For this review, take the finished solid that the model builds, in its own axes (mm). Give positions to 0.01 mm unless a question says otherwise; leave off trailing zeros. Order: outer loops, then holes, each group sorted by start corner. A loop starts at its lowest first (then second) coordinate and runs counter-clockwise, first axis right, second up. Notation, with made-up numbers: M -18,88 L 41,88 A20 cw 41,103 Z; hole C -4.5,33 d6. An arc over 180 degrees is marked long. Answer as CSV lines item,"result". Start each with the question number.
1. We need section B-B, the plane x = 0. Give the boundary of the cut face in (y, z).
2. We need section D-D, the plane y = -38. Give the boundary of the cut face in (x, z).
3. For line 1 along Z through (x, y) = (-65.5, -63.5); line 2 along X through (y, z) = (-63.5, -87); line 3 along Y through (x, z) = (0, -108), list the stretches that pass through material, from the lowest coordinate up.
4. We need section A-A, the plane z = 0. Give the boundary of the cut face in (x, y), and give its area (3 significant figures).
5. We need section C-C, the plane y = -63.5. Give the boundary of the cut face in (x, z).
from build123d import *

# Parameters (mm, degrees)
F0_W     = 254
F0_H     = 508
F1_DEPTH = 127
F3_SIZE  = 30
F4_R     = 30
F2_R     = 20
F5_DEPTH = 127.001
F6_R     = 20
F7_DEPTH = 254.001
F8_R     = 20
F9_DEPTH = 508.001


with BuildPart() as f1:
    # F0 (on Front) → F1 (new body)
    with BuildSketch(Plane.XZ):
        Rectangle(F0_W, F0_H)
    extrude(amount=F1_DEPTH)

    # F3
    f3_edges = [f1.edges().sort_by_distance(p)[0] for p in [
        (127, -63.5, 254),
        (127, -63.5, -254),
    ]]
    chamfer(f3_edges, length=F3_SIZE)

    # F4
    f4_edges = [f1.edges().sort_by_distance(p)[0] for p in [
        (-127, -63.5, 254),
        (-127, -63.5, -254),
    ]]
    fillet(f4_edges, radius=F4_R)

    # F2 (on face) → F5 (cut, through all)
    with BuildSketch(Plane.XZ.offset(127)):
        Circle(F2_R)
    extrude(amount=-F5_DEPTH, mode=Mode.SUBTRACT)

    # F6 (on face) → F7 (cut, through all)
    with BuildSketch(Plane(origin=(-127, 0, 0), x_dir=(0, -1, 0), z_dir=(-1, 0, 0))):
        with Locations((63.5, 0)):
            Circle(F6_R)
    extrude(amount=-F7_DEPTH, mode=Mode.SUBTRACT)

    # F8 (on face) → F9 (cut, through all)
    with BuildSketch(Plane.XY.offset(254)):
        with Locations((0, -63.5)):
            Circle(F8_R)
    extrude(amount=-F9_DEPTH, mode=Mode.SUBTRACT)


solid = f1.part
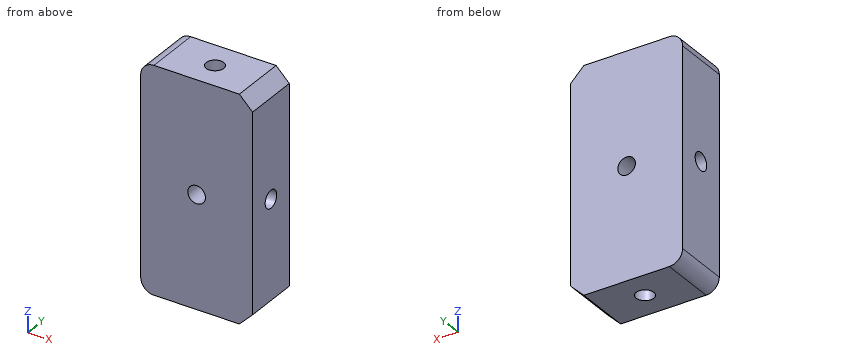
Result set:
1,outline,"M -127,-254 L -83.5,-254 L -83.5,-20 L -127,-20 Z; M -127,20 L -83.5,20 L -83.5,254 L -127,254 Z; M -43.5,-254 L 0,-254 L 0,-20 L -43.5,-20 Z; M -43.5,20 L 0,20 L 0,254 L -43.5,254 Z"
2,outline,"M -127,-224 A30 ccw -97,-254 L 97,-254 L 127,-224 L 127,224 L 97,254 L -97,254 A30 ccw -127,224 Z; hole C 0,0 d40"
3,line 1,"-254 to -20, 20 to 254"
3,line 2,"-127 to -20, 20 to 127"
3,line 3,"-127 to -83.5, -43.5 to 0"
4,outline,"M -127,-127 L -20,-127 L -20,-83.5 L -127,-83.5 Z; M -127,-43.5 L -20,-43.5 L -20,0 L -127,0 Z; M 20,-127 L 127,-127 L 127,-83.5 L 20,-83.5 Z; M 20,-43.5 L 127,-43.5 L 127,0 L 20,0 Z"
4,area,"18,600 mm2"
5,outline,"M -127,-224 A30 ccw -97,-254 L -20,-254 L -20,-20 L -127,-20 Z; M -127,20 L -20,20 L -20,254 L -97,254 A30 ccw -127,224 Z; M 20,-254 L 97,-254 L 127,-224 L 127,-20 L 20,-20 Z; M 20,20 L 127,20 L 127,224 L 97,254 L 20,254 Z"
